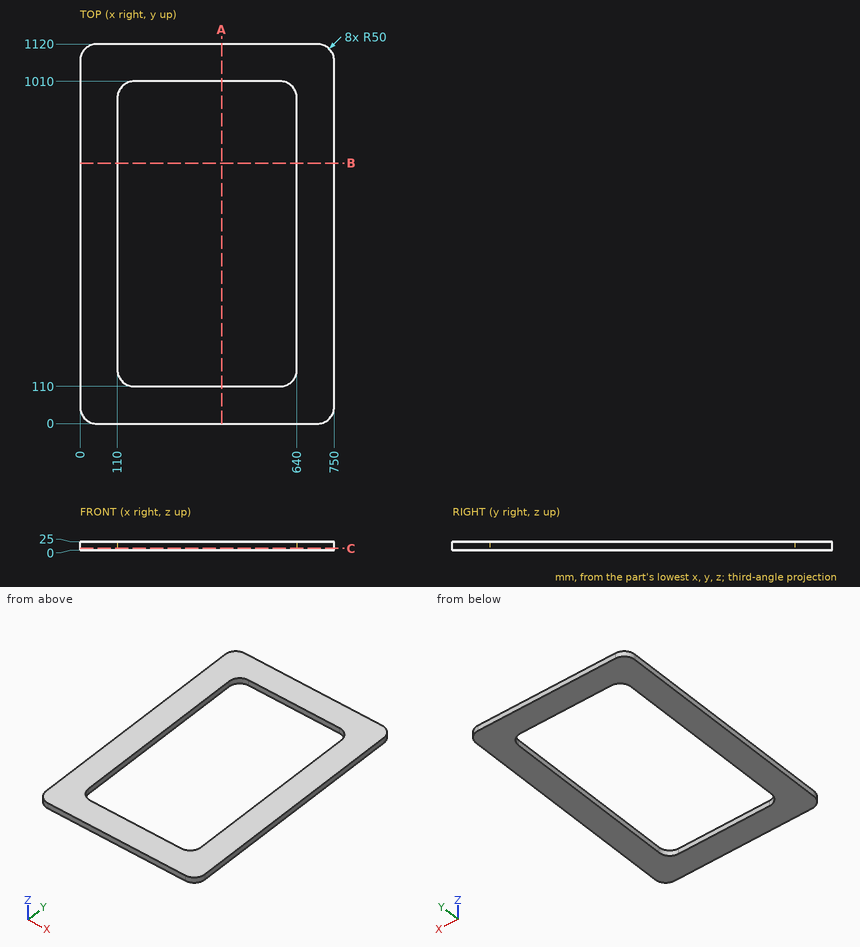
Design review of the part shown in the three views and the two pictorial views. Dimensions are in mm from the part's minimum x, y and z. Round coordinates to 2 decimals unless told otherwise and drop trailing zeros. Order: outer loops, then holes, each group sorted by start corner. A loop starts at its lowest first (then second) coordinate and runs counter-clockwise, first axis right, second up.
Q1. Wall thickness on line 1 (Y direction, x = 210, z = 9.25); line 2 (X direction, y = 614, z = 24); line 3 (Y direction, x = 153.5, z = 10.25): over which ranges is each line inside the solid? List them lowest first.
Findings below:
line 1: y = 0 to 110, 1010 to 1120
line 2: x = 0 to 110, 640 to 750
line 3: y = 0 to 110.42, 1009.58 to 1120
Q2. We need section C-C, the plane z = 5.5. Give the boundary of the cut face in (x, y).
Findings below:
outline: (0, 50) arc R50 ccw to (50, 0) - (700, 0) arc R50 ccw to (750, 50) - (750, 1070) arc R50 ccw to (700, 1120) - (50, 1120) arc R50 ccw to (0, 1070) - close; hole (110, 160) arc R50 ccw to (160, 110) - (590, 110) arc R50 ccw to (640, 160) - (640, 960) arc R50 ccw to (590, 1010) - (160, 1010) arc R50 ccw to (110, 960) - close
Q3. Insertion check: P1, Ø12.5, axis at x = 310, z = 12, coming from the -Y side. The pin has a flat end and moves straight along its axis. Give the tip position at first contact, or say it passes through.
Findings below:
P1: stops at y = 0
Q4. We need section A-A, the plane x = 417.5. Give the boundary of the cut face in (y, z), plus the area to 3 significant figures.
Findings below:
outline: (0, 0) - (110, 0) - (110, 25) - (0, 25) - close; (1010, 0) - (1120, 0) - (1120, 25) - (1010, 25) - close
area: 5,500 mm2
Q5. We need section B-B, the plane y = 769. Give the boundary of the cut face in (x, z).
Findings below:
outline: (0, 0) - (110, 0) - (110, 25) - (0, 25) - close; (640, 0) - (750, 0) - (750, 25) - (640, 25) - close
